from build123d import *

# Parameters (mm, degrees)
ESQUISSE1_R        = 1.25
ESQUISSE1_R_2      = 4
BOSS_EXTRU_1_DEPTH = 11
CONG_1_R           = 10


with BuildPart() as part:
    # Esquisse1 → Boss.-Extru.1 (new body)
    with BuildSketch(Plane.XY):
        Polygon((34.77820323, 124.002253451), (124.77820323, -31.88231923), (124.77820323, -72.040729224), (90, -92.119934221), (-90, -92.119934221), (-124.77820323, -72.040729224), (-124.77820323, -31.88231923), (-34.77820323, 124.002253451), (0, 144.081458448), align=None)
        with Locations((-117.85, -68.040729224)):
            Circle(ESQUISSE1_R, mode=Mode.SUBTRACT)
        with Locations((117.85, -68.040729224)):
            Circle(ESQUISSE1_R, mode=Mode.SUBTRACT)
        with Locations((0, 136.081458448)):
            Circle(ESQUISSE1_R, mode=Mode.SUBTRACT)
        with Locations((-86.240072762, -49.790729224)):
            Circle(ESQUISSE1_R, mode=Mode.SUBTRACT)
        with Locations((0, 99.581458448)):
            Circle(ESQUISSE1_R, mode=Mode.SUBTRACT)
        with Locations((86.240072762, -49.790729224)):
            Circle(ESQUISSE1_R, mode=Mode.SUBTRACT)
        with Locations((-61, -35.218366421)):
            Circle(ESQUISSE1_R_2, mode=Mode.SUBTRACT)
        with Locations((0, 70.436732841)):
            Circle(ESQUISSE1_R_2, mode=Mode.SUBTRACT)
        with Locations((61, -35.218366421)):
            Circle(ESQUISSE1_R_2, mode=Mode.SUBTRACT)
        with Locations((22.5, 119.800180857)):
            Circle(ESQUISSE1_R_2, mode=Mode.SUBTRACT)
        with Locations((-22.5, 119.800180857)):
            Circle(ESQUISSE1_R_2, mode=Mode.SUBTRACT)
        with Locations((-115, -40.414518843)):
            Circle(ESQUISSE1_R_2, mode=Mode.SUBTRACT)
        with Locations((-92.5, -79.385662014)):
            Circle(ESQUISSE1_R_2, mode=Mode.SUBTRACT)
        with Locations((92.5, -79.385662014)):
            Circle(ESQUISSE1_R_2, mode=Mode.SUBTRACT)
        with Locations((115, -40.414518843)):
            Circle(ESQUISSE1_R_2, mode=Mode.SUBTRACT)
    extrude(amount=BOSS_EXTRU_1_DEPTH)

    # Congé1
    cong_1_edges = [part.edges().sort_by_distance(p)[0] for p in [
        (34.77820323, 124.002253451, 5.5),
        (124.77820323, -31.88231923, 5.5),
        (124.77820323, -72.040729224, 5.5),
        (90, -92.119934221, 5.5),
        (-90, -92.119934221, 5.5),
        (-124.77820323, -72.040729224, 5.5),
        (-124.77820323, -31.88231923, 5.5),
        (-34.77820323, 124.002253451, 5.5),
        (0, 144.081458448, 5.5),
    ]]
    fillet(cong_1_edges, radius=CONG_1_R)


solid = part.part
Could you check a few things on this model? Use its own coordinates, in mm. Give positions to 0.01 mm unless a question says otherwise; leave off trailing zeros. Order: outer loops, then holes, each group sorted by start corner. A loop starts at its lowest first (then second) coordinate and runs counter-clockwise, first axis right, second up. Notation, with made-up numbers: (19.5, 3) - (27.5, 3) arc R21 ccw to (27.5, 21) - close; hole circle Ø8 at (-33.5, 55.5). An arc over 180 degrees is marked (long way). Return JSON: item names as keys, results as strings. Group by question number.
Q1. Suppose I cut it at B-B, the plane z = 4. State how many separate pieces and enclosed holes the cut face has, and give its area (3 significant figures).
Q2. Please list where these lines run through material, in increasing order: line 1 along X through (y, z) = (-41, 2); line 2 along Y through (x, z) = (-117.85, 6); line 3 along X through (y, z) = (-43.5, 9.75). Write a range as [from, to].
Q3. Suppose I cut it at C-C, the plane y = -16. Please give me the cut outline in (x, z), and give its area (3 significant figures).
Q4. Will these pins go through, and if not, where does the flat tip stop? pin 1 Ø9 at (x, y) = (0, 70.44) entering from -Z; pin 2 Ø4 at (x, z) = (58.5, 8.5) entering from +Y; pin 3 Ø5 at (x, z) = (-99, 2.5) entering from -Y.
Q5. Suppose I cut it at A-A, the plane x = -22.5. Please give me the cut outline in (y, z).
Q6. Thinking about a two-plate mould opening in Y: for faces 1 (the face through (21.633, 115.895, 5.423)), 2 (the face through (2, 1, 11)), 3 (the face through (79.167, 47.119, 5.423)), which applies, pulls with the +Y half, pulls with the -Y half, needs draft (parallel to the pull), parting line crosses it, or undercut?
Q7. Suppose I cut it at D-D, the plane x = 61. Please give me the cut outline in (y, z), and give its area (3 significant figures).
Resolved:
{
 "1": {"separate pieces": "1", "enclosed holes": "15", "area": "39,400 mm2"},
 "2": {"line 1": "x = [-124.78, -118.96], [-111.04, 111.04], [118.96, 124.78]", "line 2": "y = [-76.04, -69.29], [-66.79, -43.22], [-37.61, -19.88]", "line 3": "x = [-124.78, -117.55], [-112.45, 112.45], [117.55, 124.78]"},
 "3": {"outline": "(-115.61, 0) - (115.61, 0) - (115.61, 11) - (-115.61, 11) - close", "area": "2,540 mm2"},
 "4": {"pin 1": "stops at z = 0", "pin 2": "stops at y = 86.38", "pin 3": "stops at y = -88.37"},
 "5": {"outline": "(-92.12, 0) - (115.8, 0) - (115.8, 11) - (-92.12, 11) - close; (123.8, 0) - (131.09, 0) - (131.09, 11) - (123.8, 11) - close"},
 "6": {"face 1": "undercut", "face 2": "needs draft", "face 3": "pulls with the +Y half"},
 "7": {"outline": "(-92.12, 0) - (-39.22, 0) - (-39.22, 11) - (-92.12, 11) - close; (-31.22, 0) - (78.58, 0) - (78.58, 11) - (-31.22, 11) - close", "area": "1,790 mm2"}
}
